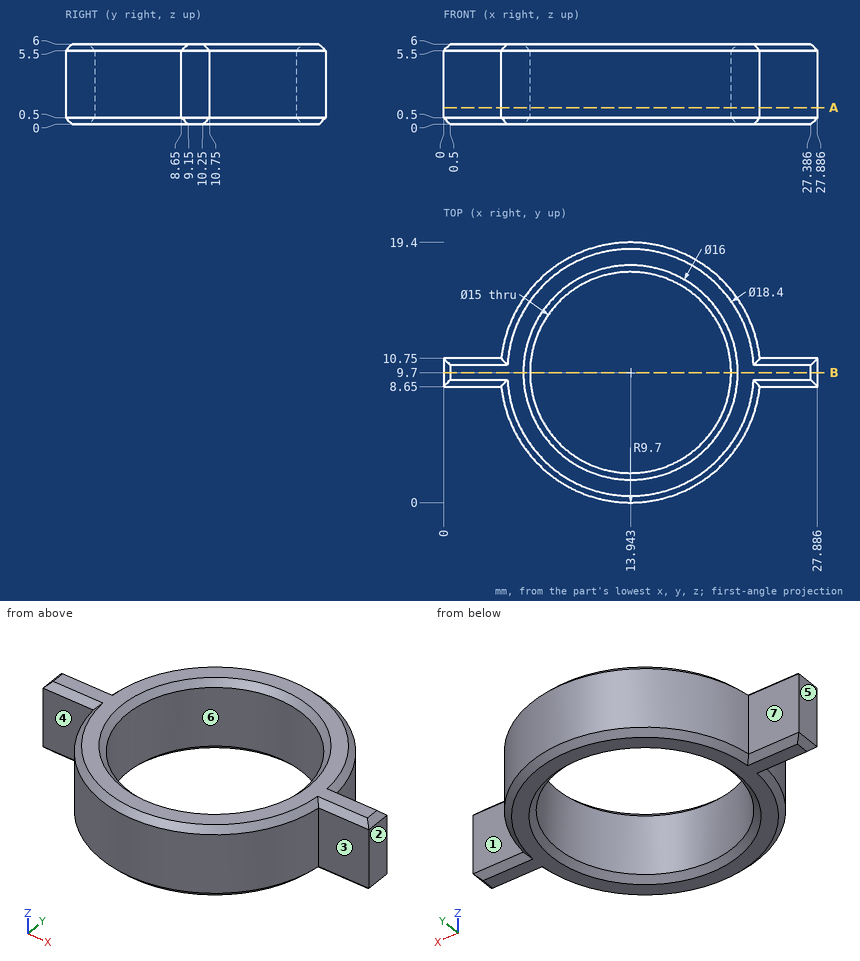
Verification items for this drawing (mm, ordinates from the low corner). A direction names the side the tool comes from. Coordinates: 2 decimals unless noted, no trailing zeros. Loops run counter-clockwise (first coordinate to the right, second up) from the corner with the lowest first, then second, coordinate; pieces in that order, holes last. Notation, with made-up numbers: (-35.5, 38) - (4.5, 38) arc R37 ccw to (4.5, 76) - close; hole circle Ø2 at (77.5, -24). An arc over 180 degrees is marked (long way). Use one line per item in the form item = value. Start each with the question number.
Item 1: Section check A-A, the plane z = 1.25. Enter the section's corners in (x, y).
Item 2: Thickness scan on probe 1 along X at (y, z) = (10, 1); probe 2 along Y at (x, z) = (11.75, 4); probe 3 along Y at (x, z) = (11, 5.25). Record the ranges inside material, lowest first.
Item 3: Mould release check, pull along Y, two halves, no side actions. Record for the marked faces 5, 6 and 7: +Y half, -Y half, draft (parallel to the pull), parting line (faces both ways), or undercut.
Item 4: Section check B-B, the plane y = 9.7. Enter the section's corners in (x, z).
Item 5: Tool access check on the marked faces 1, 2, 3 and 4. Record the directions out of +Z, -Z, +X, -X, +Y, -Y that give a thin tool (end or side, any length) a straight path to the whole face; none if there is none.
Item 6: Gauge pin test, flat ends, axial feed: pin 1 (3 mm diameter, centred on y = 14.5, z = 3, fed in from +X); pin 2 (2 mm diameter, centred on x = 2, z = 4, fed in from +Y); pin 3 (3 mm diameter, centred on x = 5, z = 4.5, fed in from -Y); pin 4 (4 mm diameter, centred on x = 21.5, y = 11, fed in from +Z). Record the tip position at first contact, or that the pin passes through.
Computed:
q1.outline = (0, 8.65) - (4.3, 8.65) arc R9.7 ccw to (23.59, 8.65) - (27.89, 8.65) - (27.89, 10.75) - (23.59, 10.75) arc R9.7 ccw to (4.3, 10.75) - (0, 10.75) - close; hole circle Ø15 at (13.94, 9.7)
q2.probe_1 = 0 to 6.45, 21.44 to 27.89
q2.probe_2 = 0.25 to 2.53, 16.87 to 19.15
q2.probe_3 = 0.46 to 2.8, 16.6 to 18.94
q3.face_5 = draft
q3.face_6 = undercut
q3.face_7 = +Y half
q4.outline = (0, 0.5) - (0.5, 0) - (5.94, 0) - (6.44, 0.5) - (6.44, 5.5) - (5.94, 6) - (0.5, 6) - (0, 5.5) - close; (21.44, 0.5) - (21.94, 0) - (27.39, 0) - (27.89, 0.5) - (27.89, 5.5) - (27.39, 6) - (21.94, 6) - (21.44, 5.5) - close
q5.face_1 = +Z, -Z, +X, +Y
q5.face_2 = +Z, -Z, +X, +Y, -Y
q5.face_3 = +Z, -Z, +X, -Y
q5.face_4 = +Z, -Z, -X, -Y
q6.pin_1 = 23.06
q6.pin_2 = 10.75
q6.pin_3 = 3.48
q6.pin_4 = 6
